Can you work these out from the model? Positions are in its coordinate system, mm. Face numbers are marked on the shaded views. Round coordinates to 2 decimals unless told otherwise and drop trailing zeros. Order: outer loops, then holes, each group sorted by start corner. A loop starts at its lowest first (then second) coordinate and runs counter-clockwise, first axis right, second up. Notation, with made-up numbers: M 86.5,-20 L 110.5,-20 A20 cw 110.5,-12 Z; hole C 42.5,56 d11. An arc over 180 degrees is marked long. One line per question, with ' | ' between items.
```python
from build123d import *

# Parameters (mm, degrees)
SKETCH_1_R          = 5
SKETCH_1_R_2        = 2.5
EXTRUDE_1_DEPTH     = 4
SKETCH_2_R          = 3.999624375
SKETCH_2_R_2        = 3.5
CUT_EXTRUDE_1_DEPTH = 0.2
SKETCH_3_R          = 3.950876812
SKETCH_3_R_2        = 3.5
CUT_EXTRUDE_2_DEPTH = 0.2
CHAMFER_1_SIZE      = 0.1


with BuildPart() as part:
    # 草图1 → 凸台-拉伸1 (new body)
    with BuildSketch(Plane(origin=(0, 0, 0), x_dir=(0, 0, -1), z_dir=(1, 0, 0))):
        Circle(SKETCH_1_R)
        Circle(SKETCH_1_R_2, mode=Mode.SUBTRACT)
    extrude(amount=EXTRUDE_1_DEPTH)

    # 草图2 → 切除-拉伸1 (cut)
    with BuildSketch(Plane(origin=(4, 0, 0), x_dir=(0, 0, -1), z_dir=(1, 0, 0))):
        with Locations((-0.000375625, 0)):
            Circle(SKETCH_2_R)
        with Locations((-0.000375625, 0)):
            Circle(SKETCH_2_R_2, mode=Mode.SUBTRACT)
    extrude(amount=-CUT_EXTRUDE_1_DEPTH, mode=Mode.SUBTRACT)

    # 草图3 → 切除-拉伸2 (cut)
    with BuildSketch(Plane.ZY):
        with Locations((-0.049123188, 0)):
            Circle(SKETCH_3_R)
        with Locations((-0.049123188, 0)):
            Circle(SKETCH_3_R_2, mode=Mode.SUBTRACT)
    extrude(amount=-CUT_EXTRUDE_2_DEPTH, mode=Mode.SUBTRACT)

    # 倒角1
    chamfer_1_edges = [part.edges().sort_by_distance(p)[0] for p in [
        (4, 0, 3.500375625),
        (0, 0, 5),
        (0, 0, -4),
        (0, 0, -3.549123188),
        (4, 0, 5),
        (0, 0, 2.5),
        (4, 0, 2.5),
    ]]
    chamfer(chamfer_1_edges, length=CHAMFER_1_SIZE)


solid = part.part
```
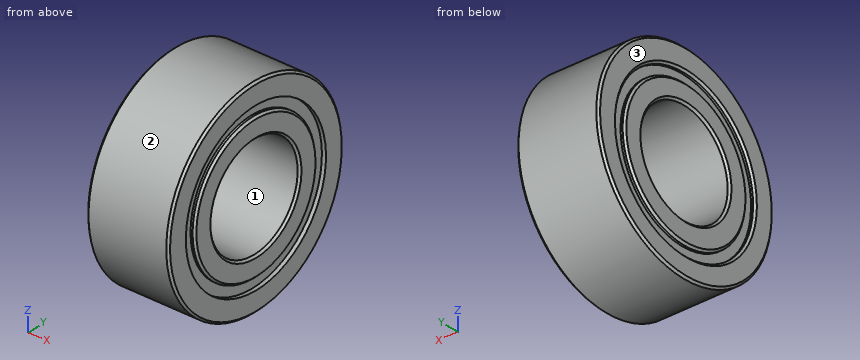
(1) Will these pins go through, and if not, where does the flat tip stop? pin 1 Ø2.5 at (y, z) = (-1, 0.5) entering from -X; pin 2 Ø1 at (x, y) = (1, 2.5) entering from -Z; pin 3 Ø1 at (x, z) = (2.5, 2.5) entering from +Y; pin 4 Ø3 at (y, z) = (-2.5, 0) entering from -X.
Final values:
pin 1: through | pin 2: z = -4.58 | pin 3: y = 4.58 | pin 4: x = 0
(2) Thinking about a two-plate mould opening in Y: for the marked faces 1, 2 and 3, which applies, released by +Y, released by -Y, zero draft, split by the parting line, or undercut?
Final values:
face 1: undercut | face 2: split by the parting line | face 3: zero draft
(3) Please list where these lines run through material, in increasing order: probe 1 along Y at (x, z) = (2.1, 0); probe 2 along Y at (x, z) = (3.85, -2.25); probe 3 along Y at (x, z) = (1.6, 1.75). Write a range as [from, to].
Final values:
probe 1: [-5, -2.5], [2.5, 5] | probe 2: [-4.47, -3.31], [-2.68, -1.09], [1.09, 2.68], [3.31, 4.47] | probe 3: [-4.68, -1.79], [1.79, 4.68]
(4) If we section it at A-A on x = 2.35: Please give me the cut outline in (y, z).
Final values:
outline: C 0,0 d10; hole C 0,0 d5
